from build123d import *

# Parameters (mm, degrees)
BOSS_EXTRUDE1_DEPTH  = 5.08
M5_CLEARANCE_HOLE1_D = 5.5
M4_CLEARANCE_HOLE1_D = 4.5


with BuildPart() as part:
    # Sketch1 → Boss-Extrude1 (new body)
    with BuildSketch(Plane.XY):
        with BuildLine():
            Line((0, 10.16), (0, -10.16))
            Line((0, -10.16), (38.1, -10.16))
            ThreePointArc((38.1, -10.16), (48.26, 0), (38.1, 10.16))
            Line((38.1, 10.16), (0, 10.16))
        make_face()
    extrude(amount=BOSS_EXTRUDE1_DEPTH)

    # M5 Clearance Hole1 (through all)
    with Locations(Plane.XY.offset(5.08)):
        with Locations((38.1, 0)):
            Hole(M5_CLEARANCE_HOLE1_D / 2)

    # M4 Clearance Hole1 (through all)
    with Locations(Plane.XY.offset(5.08)):
        with Locations((19.0499945, -0.016311357), (6.35, -0.00449174)):
            Hole(M4_CLEARANCE_HOLE1_D / 2)


solid = part.part
Can you work these out from the model? Positions are in its coordinate system, mm. Round coordinates to 2 decimals unless told otherwise and drop trailing zeros. Order: outer loops, then holes, each group sorted by start corner. A loop starts at its lowest first (then second) coordinate and runs counter-clockwise, first axis right, second up. Notation, with made-up numbers: M -5,46.25 L 9,46.25 A20 ccw 9,68.25 Z; hole C 25.25,8.5 d11. An arc over 180 degrees is marked long. Use a Markdown table: item, result.
1) Imagine slicing it at C-C (z = 3.75). List the corners of the cut face in (x, y) for me, then the cut area to 3 significant figures.
Geometry says:
| item | result |
|---|---|
| outline | M 0,-10.16 L 38.1,-10.16 A10.16 ccw 38.1,10.16 L 0,10.16 Z; hole C 6.35,0 d4.5; hole C 19.05,-0.02 d4.5; hole C 38.1,0 d5.5 |
| area | 881 mm² |
2) If I drill on line 1 along Y through (x, z) = (6.35, 2.95); line 2 along X through (y, z) = (-1.5, 4.5); line 3 along X through (y, z) = (2, 4.5), over which ranges is the centre line in solid material (lowest first)?
Geometry says:
| item | result |
|---|---|
| line 1 | y = -10.16 to -2.25, 2.25 to 10.16 |
| line 2 | x = 0 to 4.67, 8.03 to 17.36, 20.74 to 35.8, 40.4 to 48.15 |
| line 3 | x = 0 to 5.33, 7.37 to 18.05, 20.05 to 36.21, 39.99 to 48.06 |
3) Imagine slicing it at A-A (x = 6.35). List the corners of the cut face in (y, z) for me.
Geometry says:
| item | result |
|---|---|
| outline | M -10.16,0 L -2.25,0 L -2.25,5.08 L -10.16,5.08 Z; M 2.25,0 L 10.16,0 L 10.16,5.08 L 2.25,5.08 Z |
4) If we mould it in two halves opening along X, with no side actions, what happens to faces 1 (the face through (16.904, 0.66, 2.504)), 2 (the face through (4.204, 0.671, 2.504)), 3 (the face through (48.258, -0.223, 2.504)), 4 (the face through (19, 10.16, 3))? For each: +X half, -X half, draft (parallel to the pull), parting line (faces both ways), or undercut.
Geometry says:
| item | result |
|---|---|
| face 1 | undercut |
| face 2 | undercut |
| face 3 | +X half |
| face 4 | draft |
5) Imagine slicing it at D-D (x = 39.5). List the corners of the cut face in (y, z) for me, then the cut area to 3 significant figures.
Geometry says:
| item | result |
|---|---|
| outline | M -10.06,0 L -2.37,0 L -2.37,5.08 L -10.06,5.08 Z; M 2.37,0 L 10.06,0 L 10.06,5.08 L 2.37,5.08 Z |
| area | 78.2 mm² |
6) I'm going to push flat-ended pins straight in: P1, Ø7, axis at x = 38.1, y = 0, coming from the -Z side; P2, Ø4, axis at x = 19.05, y = -0.02, coming from the -Z side. Where does each tip first touch, or does it pass through?
Geometry says:
| item | result |
|---|---|
| P1 | stops at z = 0 |
| P2 | passes through |
7) Imagine slicing it at B-B (y = 0.5). List the corners of the cut face in (x, z) for me, then the cut area to 3 significant figures.
Geometry says:
| item | result |
|---|---|
| outline | M 0,0 L 4.16,0 L 4.16,5.08 L 0,5.08 Z; M 8.54,0 L 16.86,0 L 16.86,5.08 L 8.54,5.08 Z; M 21.24,0 L 35.4,0 L 35.4,5.08 L 21.24,5.08 Z; M 40.8,0 L 48.25,0 L 48.25,5.08 L 40.8,5.08 Z |
| area | 173 mm² |
